Work out the finished part from the listing and answer in its coordinate system (mm). Face numbers are marked on the shaded views. A direction names the side the tool comes from. Coordinates: 2 decimals unless noted, no trailing zeros. Loops run counter-clockwise (first coordinate to the right, second up) from the corner with the lowest first, then second, coordinate; pieces in that order, holes last. Notation, with made-up numbers: (68, 60.5) - (105, 60.5) arc R32 ccw to (105, 88.5) - close; hole circle Ø10 at (-38.75, 22.25). An arc over 180 degrees is marked (long way). Write each question's results on one line, items separated by ' | '. Start each with the question number.
1. Each of these flat-tipped pins is pushed along its axis until it touches: P1, Ø5, axis at x = 9, z = -6.5, coming from the -Y side; P2, Ø3, axis at x = 3.5, z = 3.5, coming from the -Y side; P3, Ø5, axis at y = -4, z = -1, coming from the +X side. Where does it stop, or does it pass through?
2. Determine the mould class of the marked faces 1, 2 and 3 for opening direction Z: released by +Z, released by -Z, zero draft, split by the parting line, or undercut.
3. A cutting plane is placed at B-B on x = 3. Determine the outline of the cut face in (y, z) (3 decimals), then the cut area to 3 significant figures.
4. Which of the six approach directions +Z, -Z, +X, -X, +Y, -Y give full straight-line access (tool end or side, diameter ignored) to the marked faces 4, 5 and 6?
5. A cutting plane is placed at D-D on x = 6.35. Determine the outline of the cut face in (y, z) (3 decimals), then the cut area to 3 significant figures.
6. Find the intervals of material crossed by line 1 along Z through (x, y) = (4.5, 3.25) (3 decimals); line 2 along X through (y, z) = (-2, -1.75); line 3 along X through (y, z) = (0.75, 5.75), in increasing order. Write a range as [from, to].
7. A cutting plane is placed at A-A on y = -2.5. Determine the outline of the cut face in (x, z) (3 decimals), then the cut area to 3 significant figures.
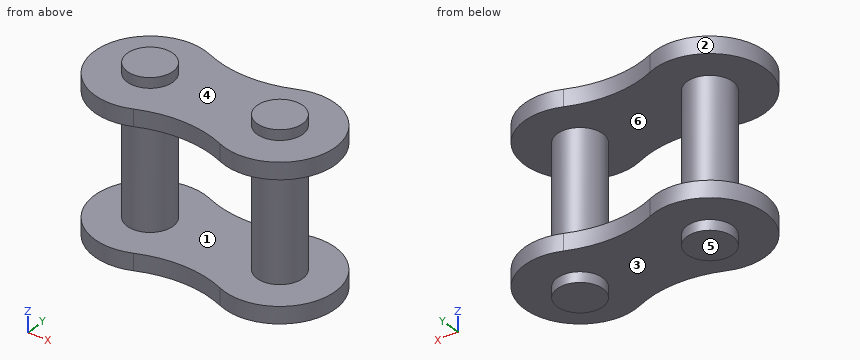
from build123d import *

# Parameters (mm, degrees)
SKETCH_1_R        = 2.23
EXTRUDE_1_DEPTH   = 8.5
EXTRUDE_1_2_DEPTH = 8.5
EXTRUDE_START     = 5.875
EXTRUDE_2_DEPTH   = 1.63


with BuildPart() as part:
    # Sketch 1 → Extrude 1 (new, symmetric)
    with BuildSketch(Plane.XY):
        with Locations((-6.35, 0)):
            Circle(SKETCH_1_R)
    extrude(amount=EXTRUDE_1_DEPTH, both=True)



with BuildPart() as body_2:
    # Sketch 1 → Extrude 1 2 (new, symmetric)
    with BuildSketch(Plane.XY):
        with Locations((6.35, 0)):
            Circle(SKETCH_1_R)
    extrude(amount=EXTRUDE_1_2_DEPTH, both=True)


with BuildPart() as part_1:
    add(part.part)

    add(body_2.part)  # Extrude 2 merges body 2
    # Sketch 2 → Extrude 2 (add)
    with BuildSketch(Plane.XY.offset(EXTRUDE_START)):
        with BuildLine():
            ThreePointArc((-4.23202836, 4.978182011), (-11.76, 0), (-4.23202836, -4.978182011))
            ThreePointArc((-4.23202836, -4.978182011), (0, -4.115344217), (4.23202836, -4.978182011))
            ThreePointArc((4.23202836, -4.978182011), (11.76, 0), (4.23202836, 4.978182011))
            ThreePointArc((4.23202836, 4.978182011), (0, 4.115344217), (-4.23202836, 4.978182011))
        make_face()
    extrude_2 = extrude(amount=EXTRUDE_2_DEPTH)

    # Mirror 1: Extrude 2 across plane
    add(extrude_2.mirror(Plane.XY))


solid = part_1.part
Values:
1) P1: y = -5.41 | P2: y = -1.77 | P3: x = 8
2) face 1: undercut | face 2: zero draft | face 3: released by -Z
3) outline: (-4.54, -7.505) - (4.54, -7.505) - (4.54, -5.875) - (-4.54, -5.875) - close; (-4.54, 5.875) - (4.54, 5.875) - (4.54, 7.505) - (-4.54, 7.505) - close | area: 29.6 mm^2
4) face 4: +Z | face 5: -Z, +X, -X, +Y, -Y | face 6: none
5) outline: (-5.41, -7.505) - (-2.23, -7.505) - (-2.23, -8.5) - (2.23, -8.5) - (2.23, -7.505) - (5.41, -7.505) - (5.41, -5.875) - (2.23, -5.875) - (2.23, 5.875) - (5.41, 5.875) - (5.41, 7.505) - (2.23, 7.505) - (2.23, 8.5) - (-2.23, 8.5) - (-2.23, 7.505) - (-5.41, 7.505) - (-5.41, 5.875) - (-2.23, 5.875) - (-2.23, -5.875) - (-5.41, -5.875) - close | area: 96.6 mm^2
6) line 1: [-7.505, -5.875], [5.875, 7.505] | line 2: [-7.34, -5.36], [5.36, 7.34] | line 3: [-8.45, -4.25], [4.25, 8.45]
7) outline: (-11.148, -7.505) - (11.148, -7.505) - (11.148, -5.875) - (-11.148, -5.875) - close; (-11.148, 5.875) - (11.148, 5.875) - (11.148, 7.505) - (-11.148, 7.505) - close | area: 72.7 mm^2
